```python
from build123d import *

# Parameters (mm, degrees)
BOSS_EXTRUDE1_DEPTH = 12.7
CUT_EXTRUDE1_DEPTH  = 314.689643597
LPATTERN1_COUNT     = 3
LPATTERN1_PITCH     = 65.7


with BuildPart() as part:
    # Sketch1 → Boss-Extrude1 (new body)
    with BuildSketch(Plane.XY):
        with BuildLine():
            Line((210.5, 170), (210.5, 0))
            Line((210.5, 0), (219.1, 0))
            ThreePointArc((219.1, 0), (222.3, 3.2), (225.5, 0))
            Line((225.5, 0), (225.5, -19.05))
            Line((225.5, -19.05), (250, -19.05))
            Line((250, -19.05), (250, 0))
            Line((250, 0), (250, 170))
            Line((250, 170), (250, 189.05))
            Line((250, 189.05), (225.5, 189.05))
            Line((225.5, 189.05), (225.5, 170))
            ThreePointArc((225.5, 170), (222.3, 166.8), (219.1, 170))
            Line((219.1, 170), (210.5, 170))
        make_face()
    extrude(amount=BOSS_EXTRUDE1_DEPTH)

    # Sketch2 → Cut-Extrude1 (cut, through all)
    with BuildSketch(Plane.XY.offset(12.7)):
        with BuildLine():
            Line((210.5, 157.2), (210.5, 170))
            Line((210.5, 170), (219.1, 170))
            ThreePointArc((219.1, 170), (222.3, 173.2), (225.5, 170))
            Line((225.5, 170), (225.5, 157.2))
            ThreePointArc((225.5, 157.2), (222.3, 154), (219.1, 157.2))
            Line((219.1, 157.2), (210.5, 157.2))
        make_face()
    cut_extrude1 = extrude(amount=-CUT_EXTRUDE1_DEPTH, mode=Mode.SUBTRACT)

    # LPattern1: Cut-Extrude1 ×3
    with Locations(*[(0, -i * LPATTERN1_PITCH, 0) for i in range(1, LPATTERN1_COUNT)]):
        add(cut_extrude1, mode=Mode.SUBTRACT)


solid = part.part
```
Can you work these out from the model? Positions are in its coordinate system, mm. A direction names the side the tool comes from. Coordinates: 2 decimals unless noted, no trailing zeros. Loops run counter-clockwise (first coordinate to the right, second up) from the corner with the lowest first, then second, coordinate; pieces in that order, holes last. Notation, with made-up numbers: M 66,1 L 73,1 A31 ccw 73,37 Z; hole C -32.75,55.5 d8. An arc over 180 degrees is marked long. Put each result on its own line as item: value. Start each with the question number.
(1) Which directions (+Z, -Z, +X, -X, +Y, -Y) give clear straight access to the entire face, cutting with the end or side of a thin tool? Please do faces 1 (the face through (225.5, 32, 6)), 2 (the face through (222.4, 22.6, 6.4)), 3 (the face through (215, 157.2, 6)).
(2) Imagine slicing it at C-C on y = 163.5. List the corners of the cut face in (x, z) for me.
(3) I need wall thicknesses on probe 1 along Y at (x, z) = (214.5, 10); probe 2 along Y at (x, z) = (225, 2.5); probe 3 along X at (y, z) = (99.5, 4). Which ranges of each line are inside material? Lowest first, please.
(4) Imagine slicing it at A-A on x = 222.3. List the corners of the cut face in (y, z) for me, and give its area (3 significant figures).
(5) We'd pull the mould along Y, two halves only. Please class faces 4 (the face through (215, 0, 6)), 5 (the face through (222.4, 88.3, 6.4)), 6 (the face through (230, 86, 0)): +Y half, -Y half, draft (parallel to the pull), parting line (faces both ways), or undercut.
(6) Imagine slicing it at B-B on z = 6.25. List the corners of the cut face in (x, y) for me, and give its area (3 significant figures).
(7) Will these pins go through, and if not, where does the flat tip stop? pin 1 Ø7 at (x, z) = (215, 5) entering from -Y; pin 2 Ø2.5 at (x, z) = (213, 5) entering from +Y; pin 3 Ø6.5 at (y, z) = (172.5, 4) entering from -X.
Worked answers:
1. face 1: +Z, -Z, -X
1. face 2: +Z, -Z
1. face 3: +Z, -Z, -X, +Y
2. outline: M 225.5,0 L 250,0 L 250,12.7 L 225.5,12.7 Z
3. probe 1: y = 0 to 25.8, 38.6 to 91.5, 104.3 to 157.2
3. probe 2: y = 1.72 to 24.08, 40.32 to 89.78, 106.02 to 155.48
3. probe 3: x = 225.5 to 250
4. outline: M 3.2,0 L 22.6,0 L 22.6,12.7 L 3.2,12.7 Z; M 41.8,0 L 88.3,0 L 88.3,12.7 L 41.8,12.7 Z; M 107.5,0 L 154,0 L 154,12.7 L 107.5,12.7 Z
4. area: 1,430 mm2
5. face 4: -Y half
5. face 5: undercut
5. face 6: draft
6. outline: M 210.5,0 L 219.1,0 A3.2 cw 225.5,0 L 225.5,-19.05 L 250,-19.05 L 250,189.05 L 225.5,189.05 L 225.5,157.2 A3.2 cw 219.1,157.2 L 210.5,157.2 L 210.5,104.3 L 219.1,104.3 A3.2 cw 225.5,104.3 L 225.5,91.5 A3.2 cw 219.1,91.5 L 210.5,91.5 L 210.5,38.6 L 219.1,38.6 A3.2 cw 225.5,38.6 L 225.5,25.8 A3.2 cw 219.1,25.8 L 210.5,25.8 Z
6. area: 6,980 mm2
7. pin 1: stops at y = 0
7. pin 2: stops at y = 157.2
7. pin 3: stops at x = 225.5
